The listing builds one solid part. Answer for the finished solid, in the listing's coordinates (mm). A direction names the side the tool comes from. Round coordinates to 2 decimals unless told otherwise and drop trailing zeros. Loops run counter-clockwise (first coordinate to the right, second up) from the corner with the lowest first, then second, coordinate; pieces in that order, holes last. Notation, with made-up numbers: (35, 50) - (55, 50) arc R25 ccw to (55, 68) - close; hole circle Ø6 at (60, -14). An arc over 180 degrees is marked (long way). One line per question, with ' | ' between items. Start each with the question number.
from build123d import *

# Parameters (mm, degrees)
BOSS_EXTRUDE1_DEPTH = 1
CUT_EXTRUDE1_REACH  = 93.929
SKETCH2_R           = 3
SKETCH3_R           = 4
SKETCH3_R_2         = 3
BOSS_EXTRUDE2_DEPTH = 15
BOSS_EXTRUDE3_START = -2
SKETCH4_R           = 3
SKETCH4_R_2         = 1.5
BOSS_EXTRUDE3_DEPTH = 2
BOSS_EXTRUDE4_DEPTH = 15
SKETCH8_R           = 34
SKETCH8_R_2         = 33
SKETCH8_R_3         = 26.25
SKETCH8_R_4         = 25
BOSS_EXTRUDE5_DEPTH = 3
BOSS_EXTRUDE6_START = -1
SKETCH9_R           = 34
BOSS_EXTRUDE6_DEPTH = 1
SKETCH10_R          = 33
SKETCH10_R_2        = 26.25
CUT_EXTRUDE6_DEPTH  = 1


with BuildPart() as part:
    # Sketch1 → Boss-Extrude1 (new body)
    with BuildSketch(Plane(origin=(0, 0, 0), x_dir=(1, 0, 0), z_dir=(0, 1, 0))):
        with BuildLine():
            Line((61.02, 46.990674783), (-44.909648, 46.990674783))
            ThreePointArc((-44.909648, 46.990674783), (-35.615966741, -54.373733669), (61.02, -22.395526339))
            Line((61.02, -22.395526339), (61.02, 46.990674783))
        make_face()
    extrude(amount=BOSS_EXTRUDE1_DEPTH)

    # Sketch2 → Cut-Extrude1 (cut, up to next)
    with BuildSketch(Plane(origin=(0, 1, 0), x_dir=(1, 0, 0), z_dir=(0, 1, 0)), mode=Mode.PRIVATE) as cut_extrude1_sk1:
        with Locations(Location((-41.909648, 41.990674783, 0), (0, 0, 270))):
            Circle(SKETCH2_R)
    cut_extrude1_tool1 = extrude(cut_extrude1_sk1.sketch, amount=-CUT_EXTRUDE1_REACH, mode=Mode.PRIVATE) & part.part
    # Sketch2 → Cut-Extrude1 (cut, up to next)
    with BuildSketch(Plane(origin=(0, 1, 0), x_dir=(1, 0, 0), z_dir=(0, 1, 0)), mode=Mode.PRIVATE) as cut_extrude1_sk2:
        with Locations(Location((56.02, 41.990674783, 0), (0, 0, 270))):
            Circle(SKETCH2_R)
    cut_extrude1_tool2 = extrude(cut_extrude1_sk2.sketch, amount=-CUT_EXTRUDE1_REACH, mode=Mode.PRIVATE) & part.part
    # Sketch2 → Cut-Extrude1 (cut, up to next)
    with BuildSketch(Plane(origin=(0, 1, 0), x_dir=(1, 0, 0), z_dir=(0, 1, 0)), mode=Mode.PRIVATE) as cut_extrude1_sk3:
        with Locations(Location((40.5, -43.009325217, 0), (0, 0, 270))):
            Circle(SKETCH2_R)
    cut_extrude1_tool3 = extrude(cut_extrude1_sk3.sketch, amount=-CUT_EXTRUDE1_REACH, mode=Mode.PRIVATE) & part.part
    # Sketch2 → Cut-Extrude1 (cut, up to next)
    with BuildSketch(Plane(origin=(0, 1, 0), x_dir=(1, 0, 0), z_dir=(0, 1, 0)), mode=Mode.PRIVATE) as cut_extrude1_sk4:
        with Locations(Location((-33.98, -47.009325217, 0), (0, 0, 270))):
            Circle(SKETCH2_R)
    cut_extrude1_tool4 = extrude(cut_extrude1_sk4.sketch, amount=-CUT_EXTRUDE1_REACH, mode=Mode.PRIVATE) & part.part
    add(cut_extrude1_tool1.solids().sort_by_distance((-41.909648, 1, -41.990675))[0], mode=Mode.SUBTRACT)
    add(cut_extrude1_tool2.solids().sort_by_distance((56.02, 1, -41.990675))[0], mode=Mode.SUBTRACT)
    add(cut_extrude1_tool3.solids().sort_by_distance((40.5, 1, 43.009325))[0], mode=Mode.SUBTRACT)
    add(cut_extrude1_tool4.solids().sort_by_distance((-33.98, 1, 47.009325))[0], mode=Mode.SUBTRACT)

    # Sketch3 → Boss-Extrude2 (add)
    # profile 1 of 4: a face of its own
    with BuildSketch(Plane.XZ):
        with Locations(Location((56.02, -41.990674783, 0), (0, 0, 90))):
            Circle(SKETCH3_R)
        with Locations(Location((56.02, -41.990674783, 0), (0, 0, 90))):
            Circle(SKETCH3_R_2, mode=Mode.SUBTRACT)
    # profile 2 of 4: a face of its own
    with BuildSketch(Plane.XZ):
        with Locations(Location((-41.909648, -41.990674783, 0), (0, 0, 90))):
            Circle(SKETCH3_R)
        with Locations(Location((-41.909648, -41.990674783, 0), (0, 0, 90))):
            Circle(SKETCH3_R_2, mode=Mode.SUBTRACT)
    # profile 3 of 4: a face of its own
    with BuildSketch(Plane.XZ):
        with Locations(Location((40.5, 43.009325217, 0), (0, 0, 90))):
            Circle(SKETCH3_R)
        with Locations(Location((40.5, 43.009325217, 0), (0, 0, 90))):
            Circle(SKETCH3_R_2, mode=Mode.SUBTRACT)
    # profile 4 of 4: a face of its own
    with BuildSketch(Plane.XZ):
        with Locations(Location((-33.98, 47.009325217, 0), (0, 0, 90))):
            Circle(SKETCH3_R)
        with Locations(Location((-33.98, 47.009325217, 0), (0, 0, 90))):
            Circle(SKETCH3_R_2, mode=Mode.SUBTRACT)
    extrude(amount=BOSS_EXTRUDE2_DEPTH)

    # Sketch4 → Boss-Extrude3 (add)
    # profile 1 of 4: a face of its own
    with BuildSketch(Plane.XZ.offset(15).offset(BOSS_EXTRUDE3_START)):
        with Locations(Location((56.02, -41.990674783, 0), (0, 0, 90))):
            Circle(SKETCH4_R)
        with Locations(Location((56.02, -41.990674783, 0), (0, 0, 270))):
            Circle(SKETCH4_R_2, mode=Mode.SUBTRACT)
    # profile 2 of 4: a face of its own
    with BuildSketch(Plane.XZ.offset(15).offset(BOSS_EXTRUDE3_START)):
        with Locations(Location((-41.909648, -41.990674783, 0), (0, 0, 90))):
            Circle(SKETCH4_R)
        with Locations(Location((-41.909648, -41.990674783, 0), (0, 0, 270))):
            Circle(SKETCH4_R_2, mode=Mode.SUBTRACT)
    # profile 3 of 4: a face of its own
    with BuildSketch(Plane.XZ.offset(15).offset(BOSS_EXTRUDE3_START)):
        with Locations(Location((-33.98, 47.009325217, 0), (0, 0, 90))):
            Circle(SKETCH4_R)
        with Locations(Location((-33.98, 47.009325217, 0), (0, 0, 270))):
            Circle(SKETCH4_R_2, mode=Mode.SUBTRACT)
    # profile 4 of 4: a face of its own
    with BuildSketch(Plane.XZ.offset(15).offset(BOSS_EXTRUDE3_START)):
        with Locations(Location((40.5, 43.009325217, 0), (0, 0, 90))):
            Circle(SKETCH4_R)
        with Locations(Location((40.5, 43.009325217, 0), (0, 0, 270))):
            Circle(SKETCH4_R_2, mode=Mode.SUBTRACT)
    extrude(amount=BOSS_EXTRUDE3_DEPTH)

    # Sketch5 → Boss-Extrude4 (add)
    with BuildSketch(Plane.XZ):
        with BuildLine():
            Line((61.02, -46.990674783), (-44.909648, -46.990674783))
            ThreePointArc((-44.909648, -46.990674783), (-35.615966741, 54.373733669), (61.02, 22.395526339))
            Line((61.02, 22.395526339), (61.02, -46.990674783))
        make_face()
        with BuildLine():
            Line((-38.445546385, -43.990674783), (52.555898385, -43.990674783))
            ThreePointArc((52.555898385, -43.990674783), (58.848427125, -44.819101907), (58.02, -38.526573168))
            Line((58.02, -38.526573168), (58.02, 21.855882503))
            ThreePointArc((58.02, 21.855882503), (52.354897092, 33.210913123), (44.496580109, 43.174695814))
            ThreePointArc((44.496580109, 43.174695814), (43.242199594, 45.921427789), (40.425106883, 47.008624034))
            ThreePointArc((40.425106883, 47.008624034), (2.711724037, 61.940669618), (-36.162300139, 50.361573136))
            ThreePointArc((-36.162300139, 50.361573136), (-36.323268199, 50.25109852), (-36.478654103, 50.132901321))
            ThreePointArc((-36.478654103, 50.132901321), (-61.676302569, 6.327219087), (-45.897728888, -41.682112265))
            ThreePointArc((-45.897728888, -41.682112265), (-43.093288061, -45.811538063), (-38.445546385, -43.990674783))
        make_face(mode=Mode.SUBTRACT)
    extrude(amount=BOSS_EXTRUDE4_DEPTH)

    # Sketch8 → Boss-Extrude5 (add)
    # profile 1 of 2: a face of its own
    with BuildSketch(Plane(origin=(0, 0, 0), x_dir=(1, 0, 0), z_dir=(0, 1, 0))):
        with Locations(Location((0, 0, 0), (0, 0, 90))):
            Circle(SKETCH8_R)
        with Locations(Location((0, 0, 0), (0, 0, 270))):
            Circle(SKETCH8_R_2, mode=Mode.SUBTRACT)
    # profile 2 of 2: a face of its own
    with BuildSketch(Plane(origin=(0, 0, 0), x_dir=(1, 0, 0), z_dir=(0, 1, 0))):
        with Locations(Location((0, 0, 0), (0, 0, 90))):
            Circle(SKETCH8_R_3)
        with Locations(Location((0, 0, 0), (0, 0, 270))):
            Circle(SKETCH8_R_4, mode=Mode.SUBTRACT)
    extrude(amount=-BOSS_EXTRUDE5_DEPTH)

    # Sketch9 → Boss-Extrude6 (add)
    with BuildSketch(Plane.XZ.offset(3).offset(BOSS_EXTRUDE6_START)):
        with Locations(Location((0, 0, 0), (0, 0, 270))):
            Circle(SKETCH9_R)
    extrude(amount=BOSS_EXTRUDE6_DEPTH)

    # Sketch10 → Cut-Extrude6 (cut)
    with BuildSketch(Plane(origin=(0, 1, 0), x_dir=(1, 0, 0), z_dir=(0, 1, 0))):
        with Locations(Location((0, 0, 0), (0, 0, 270))):
            Circle(SKETCH10_R)
        with Locations(Location((0, 0, 0), (0, 0, 270))):
            Circle(SKETCH10_R_2, mode=Mode.SUBTRACT)
    extrude(amount=-CUT_EXTRUDE6_DEPTH, mode=Mode.SUBTRACT)


solid = part.part
(1) Find section D-D on x = -55.5. Write down the section's boundary in (y, z), plus the area to 3 significant figures.
(2) Determine the mould class of faces 1 (the flat face through (-2.9, 1, 33.1)), 2 (the flat face through (9, -7, -46.991)), 3 (the flat face through (-40.6, -13, -40.7)) for opening direction Z: pulls with the +Z half, pulls with the -Z half, needs draft (parallel to the pull), parting line crosses it, or undercut.
(3) Find section B-B on x = 0. Write down the section's boundary in (y, z), plus the area to 3 significant figures.
(4) Find section C-C on y = -5.75. Write down the section's boundary in (x, z).
(5) Each of these flat-tipped pins is pushed along its axis until it touches: P1, Ø1.8, axis at x = 55.5, z = -42, coming from the +Y side; P2, Ø1, axis at y = -8, z = 44, coming from the +X side; P3, Ø1.5, axis at y = -11, z = 21.5, coming from the -X side; P4, Ø3, axis at x = -34, z = 46, coming from the +Y side. Where does it stop, or does it pass through?
(6) Consider L1, parallel to Y at x = 3.5, z = -5; L2, parallel to X at y = -7, z = 40.5 (3 decimals); L3, parallel to X at y = -2.5, z = 45.5. Determine where each line is inside the solid, lowest interval first.
(7) A tool of negligible diameter and unlimited length cuts with its end or side. For faces 4 (the cylindrical face through (7.509, -0.986, 23.846)), 5 (the flat face through (57.3, -13, -40.7)), 6 (the flat face through (0, -3, 0)), 7 (the flat face through (3, -15, -45)), from which of +Z, -Z, +X, -X, +Y, -Y can it reach the whole face along a straight path? Write none if from no direction.
(8) Find section A-A on z = 0. Write down the section's boundary in (x, y), plus the area to 3 significant figures.
Answer below:
1) outline: (-15, -33.83) - (1, -33.83) - (1, 33.83) - (-15, 33.83) - (-15, 27.64) - (0, 27.64) - (0, -27.64) - (-15, -27.64) - close | area: 254 mm2
2) face 1: needs draft | face 2: pulls with the -Z half | face 3: undercut
3) outline: (-15, -46.99) - (1, -46.99) - (1, -33) - (-2, -33) - (-2, -26.25) - (1, -26.25) - (1, 26.25) - (-2, 26.25) - (-2, 33) - (1, 33) - (1, 65) - (-15, 65) - (-15, 62) - (0, 62) - (0, 34) - (-3, 34) - (-3, -34) - (0, -34) - (0, -43.99) - (-15, -43.99) - close; hole (-2, -25) - (0, -25) - (0, 25) - (-2, 25) - close | area: 265 mm2
4) outline: (-44.91, -46.99) - (61.02, -46.99) - (61.02, 22.4) arc R65 ccw (long way) to start; hole (-45.9, -41.68) arc R4 cw (long way) to (-38.45, -43.99) - (52.56, -43.99) arc R4 cw to (58.02, -38.53) - (58.02, 21.86) arc R62 ccw to (44.5, 43.17) arc R4 cw (long way) to (40.43, 47.01) arc R62 ccw to (-36.16, 50.36) arc R4 cw (long way) to (-36.48, 50.13) arc R62 ccw to start; hole circle Ø6 at (-41.91, -41.99); hole circle Ø6 at (-33.98, 47.01); hole circle Ø6 at (40.5, 43.01); hole circle Ø6 at (56.02, -41.99)
5) P1: through | P2: x = 48.3 | P3: x = -61.6 | P4: y = -13
6) L1: -3 to -2, 0 to 1 | L2: -50.84 to -46.944, 37.385 to 38.856, 42.144 to 43.615, 46.944 to 50.84 | L3: -46.42 to -42.12, -37.68 to -36.57, -31.39 to -30.28, 37.37 to 38.83, 42.17 to 46.42
7) face 4: none | face 5: +Y | face 6: -Y | face 7: +Z, -Z, +X, -X, -Y
8) outline: (-65, -15) - (-62, -15) - (-62, 0) - (-34, 0) - (-34, -3) - (34, -3) - (34, 0) - (58.02, 0) - (58.02, -15) - (61.02, -15) - (61.02, 1) - (33, 1) - (33, -2) - (26.25, -2) - (26.25, 1) - (-26.25, 1) - (-26.25, -2) - (-33, -2) - (-33, 1) - (-65, 1) - close; hole (-25, -2) - (25, -2) - (25, 0) - (-25, 0) - close | area: 280 mm2
